from build123d import *

# Parameters (mm, degrees)
SKETCH2_W           = 30
SKETCH2_H           = 6
BOSS_EXTRUDE1_DEPTH = 160
SKETCH3_R           = 1.5
CUT_EXTRUDE3_DEPTH  = 161.813556642


with BuildPart() as part:
    # Sketch2 → Boss-Extrude1 (new body)
    with BuildSketch(Plane.XY):
        Rectangle(SKETCH2_W, SKETCH2_H)
    extrude(amount=BOSS_EXTRUDE1_DEPTH)

    # Sketch3 → Cut-Extrude3 (cut, through all)
    with BuildSketch(Plane(origin=(0, 3, 0), x_dir=(1, 0, 0), z_dir=(0, 1, 0))):
        with Locations(Location((-5, -115, 0), (0, 0, 270))):
            Circle(SKETCH3_R)
        with Locations(Location((5, -115, 0), (0, 0, 270))):
            Circle(SKETCH3_R)
        with Locations(Location((5, -95, 0), (0, 0, 270))):
            Circle(SKETCH3_R)
        with Locations(Location((-5, -95, 0), (0, 0, 270))):
            Circle(SKETCH3_R)
        with Locations(Location((-5, -65, 0), (0, 0, 90))):
            Circle(SKETCH3_R)
        with Locations(Location((5, -65, 0), (0, 0, 90))):
            Circle(SKETCH3_R)
        with Locations(Location((5, -45, 0), (0, 0, 90))):
            Circle(SKETCH3_R)
        with Locations(Location((-5, -45, 0), (0, 0, 90))):
            Circle(SKETCH3_R)
    extrude(amount=-CUT_EXTRUDE3_DEPTH, mode=Mode.SUBTRACT)


solid = part.part
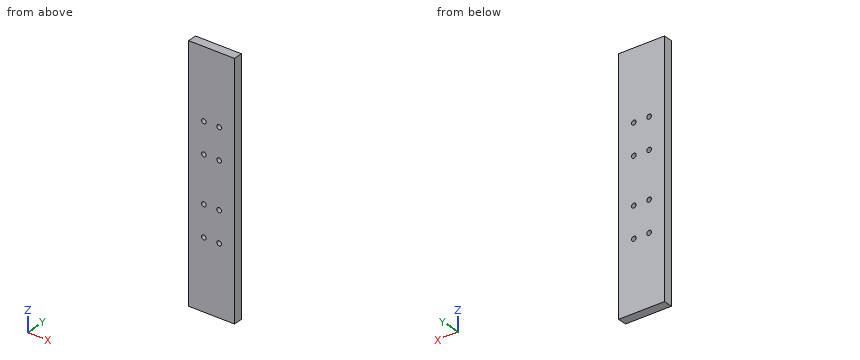
Build history of the part. All positions in model axes, mm. Give positions to 0.01 mm unless a question says otherwise; leave off trailing zeros. Order: outer loops, then holes, each group sorted by start corner. A loop starts at its lowest first (then second) coordinate and runs counter-clockwise, first axis right, second up. Notation, with made-up numbers: M 25,47 L 84,47 A27 cw 84,71 Z; hole C 60.25,-12.75 d5. An arc over 180 degrees is marked long. Put each result on its own line as item: value.
Item 1: Flat gauge pin, fed straight in: pin 1 Ø2.5 at (x, z) = (5, 65) entering from -Y. Where does the tip first touch, or does it go through?
From the geometry:
pin 1: passes through
Item 2: Probe line 1 (X direction, y = 1.65, z = 45); line 2 (Z direction, x = -6, y = 2); line 3 (X direction, y = 0.7, z = 114.5). List the from-to ranges inside material, lowest first. Write a range as [from, to].
From the geometry:
line 1: x = [-15, -6.5], [-3.5, 3.5], [6.5, 15]
line 2: z = [0, 43.88], [46.12, 63.88], [66.12, 93.88], [96.12, 113.88], [116.12, 160]
line 3: x = [-15, -6.41], [-3.59, 3.59], [6.41, 15]
Item 3: Slice it at B-B, the plane x = 5. Write the cut outline in (y, z), plus the area to 3 significant figures.
From the geometry:
outline: M -3,0 L 3,0 L 3,43.5 L -3,43.5 Z; M -3,46.5 L 3,46.5 L 3,63.5 L -3,63.5 Z; M -3,66.5 L 3,66.5 L 3,93.5 L -3,93.5 Z; M -3,96.5 L 3,96.5 L 3,113.5 L -3,113.5 Z; M -3,116.5 L 3,116.5 L 3,160 L -3,160 Z
area: 888 mm2
Item 4: Slice it at A-A, the plane z = 115. Write the cut outline in (x, y), plus the area to 3 significant figures.
From the geometry:
outline: M -15,-3 L -6.5,-3 L -6.5,3 L -15,3 Z; M -3.5,-3 L 3.5,-3 L 3.5,3 L -3.5,3 Z; M 6.5,-3 L 15,-3 L 15,3 L 6.5,3 Z
area: 144 mm2
